from build123d import *

# Parameters (mm, degrees)
SKETCH_1_W                 = 50
SKETCH_1_H                 = 45
EXTRUDE_1_DEPTH            = 12
SHELL_1_T                  = -3
SHELL_1_THICKNESS_2_FACE_W = 39
SHELL_1_THICKNESS_2_FACE_H = 44
SHELL_1_THICKNESS_2_DEPTH  = 3
HOLE_WIZARD_1_AT_2_COUNT   = 2
HOLE_WIZARD_1_AT_2_PITCH   = 35
HOLE_WIZARD_1_AT_3_COUNT   = 2
HOLE_WIZARD_1_AT_3_PITCH   = 46.097722286
HOLE_WIZARD_1_AT_4_COUNT   = 2
HOLE_WIZARD_1_AT_4_PITCH   = 30
CUT_EXTRUDE_START          = -40
SKETCH_4_W                 = 18
SKETCH_4_H                 = 6
CUT_EXTRUDE_1_DEPTH        = 12
SKETCH_5_W                 = 44
SKETCH_5_H                 = 6
CUT_EXTRUDE_2_DEPTH        = 12
SKETCH_6_W                 = 26
SKETCH_6_H                 = 12
CUT_EXTRUDE_3_DEPTH        = 12


with BuildPart() as part:
    # 草图1 → 凸台-拉伸1 (new body)
    with BuildSketch(Plane(origin=(0, 0, 0), x_dir=(1, 0, 0), z_dir=(0, 1, 0))):
        Rectangle(SKETCH_1_W, SKETCH_1_H)
    extrude(amount=EXTRUDE_1_DEPTH)

    # 抽壳1
    shell_1_openings = [part.faces().sort_by_distance(p)[0] for p in [
        (0, 12, 0),
    ]]
    offset(amount=SHELL_1_T, openings=shell_1_openings, kind=Kind.INTERSECTION)

    # 抽壳1 thickness 2 face (on inner face of the shell) → 抽壳1 thickness 2 (add)
    with BuildSketch(Plane(origin=(0, 3, 0), x_dir=(0, 0, -1), z_dir=(0, -1, 0))):
        Rectangle(SHELL_1_THICKNESS_2_FACE_W, SHELL_1_THICKNESS_2_FACE_H)
    extrude(amount=-SHELL_1_THICKNESS_2_DEPTH)

    # 草图3 → 打孔尺寸(%根据)内六角圆柱头螺钉的类型1 (revolve, cut)
    with BuildSketch(Plane(origin=(-17.5, 0, 15), x_dir=(0, 0, -1), z_dir=(1, 0, 0))):
        Polygon((0, 0), (0, 12), (1.8, 12), (1.8, 3.4), (3, 3.4), (3, 0.025), (3.025, 0), align=None)
    hole_wizard_1 = revolve(axis=Axis((-17.5, -6.35, 15), (0, 1, 0)), mode=Mode.SUBTRACT)

    # 打孔尺寸(%根据)内六角圆柱头螺钉的类型1 at 2: 打孔尺寸(%根据)内六角圆柱头螺钉的类型1 ×2
    with Locations(*[(i * HOLE_WIZARD_1_AT_2_PITCH, 0, 0) for i in range(1, HOLE_WIZARD_1_AT_2_COUNT)]):
        add(hole_wizard_1, mode=Mode.SUBTRACT)

    # 打孔尺寸(%根据)内六角圆柱头螺钉的类型1 at 3: 打孔尺寸(%根据)内六角圆柱头螺钉的类型1 ×2
    with Locations(*[Vector(0.7592566023652966, 0, -0.6507913734559685) * (i * HOLE_WIZARD_1_AT_3_PITCH) for i in range(1, HOLE_WIZARD_1_AT_3_COUNT)]):
        add(hole_wizard_1, mode=Mode.SUBTRACT)

    # 打孔尺寸(%根据)内六角圆柱头螺钉的类型1 at 4: 打孔尺寸(%根据)内六角圆柱头螺钉的类型1 ×2
    with Locations(*[(0, 0, -i * HOLE_WIZARD_1_AT_4_PITCH) for i in range(1, HOLE_WIZARD_1_AT_4_COUNT)]):
        add(hole_wizard_1, mode=Mode.SUBTRACT)

    # 草图4 → 切除-拉伸1 (cut)
    with BuildSketch(Plane.XY.offset(22.5).offset(CUT_EXTRUDE_START)):
        with Locations((4, 9)):
            Rectangle(SKETCH_4_W, SKETCH_4_H)
    extrude(amount=-CUT_EXTRUDE_1_DEPTH, mode=Mode.SUBTRACT)

    # 草图5 → 切除-拉伸2 (cut)
    with BuildSketch(Plane.XY.offset(22.5)):
        with Locations((0, 9)):
            Rectangle(SKETCH_5_W, SKETCH_5_H)
    extrude(amount=-CUT_EXTRUDE_2_DEPTH, mode=Mode.SUBTRACT)

    # 草图6 → 切除-拉伸3 (cut)
    with BuildSketch(Plane(origin=(0, 6, 0), x_dir=(1, 0, 0), z_dir=(0, 1, 0))):
        with Locations((-9, -16.5)):
            Rectangle(SKETCH_6_W, SKETCH_6_H)
    extrude(amount=-CUT_EXTRUDE_3_DEPTH, mode=Mode.SUBTRACT)


solid = part.part
Can you work these out from the model? Positions are in its coordinate system, mm. A direction names the side the tool comes from. Give positions to 0.01 mm unless a question says otherwise; leave off trailing zeros. Loops run counter-clockwise (first coordinate to the right, second up) from the corner with the lowest first, then second, coordinate; pieces in that order, holes last. Notation, with made-up numbers: (70.25, 28) -> (96.25, 28) arc R13 cw to (96.25, 45) -> close; hole circle Ø1 at (24.5, -25). An arc over 180 degrees is marked (long way). Return JSON: item names as keys, results as strings.
Q1. I want a section at B-B, the plane z = 15. List the corners of the cut face in (x, y) for me (3 decimals).
Checks:
{"outline": "(-25, 0) -> (-22, 0) -> (-22, 12) -> (-25, 12) -> close; (4, 0) -> (14.475, 0) -> (14.5, 0.025) -> (14.5, 3.4) -> (15.7, 3.4) -> (15.7, 6) -> (4, 6) -> close; (19.3, 3.4) -> (20.5, 3.4) -> (20.5, 0.025) -> (20.525, 0) -> (25, 0) -> (25, 12) -> (22, 12) -> (22, 6) -> (19.3, 6) -> close"}
Q2. I need wall thicknesses on probe 1 along Z at (x, y) = (17.5, 5.5); probe 2 along X at (y, z) = (4.85, -15); probe 3 along Z at (x, y) = (17.5, 1.5). Which ranges of each line are inside material? Lowest first, please.
Checks:
{"probe 1": "z = -22.5 to -16.8, -13.2 to 13.2, 16.8 to 22.5", "probe 2": "x = -25 to -19.3, -15.7 to 15.7, 19.3 to 25", "probe 3": "z = -22.5 to -18, -12 to 12, 18 to 22.5"}
Q3. On a 3-axis mill with a long thin cutter (end or side, diameter ignored), from which of +Z, -Z, +X, -X, +Y, -Y can I reach the whole of each face in a straight line? I mean faces 4 (the face through (-15.7, 1.7, -12.6)), 5 (the face through (13, 9, -21)), 6 (the face through (-22.5, 12, -5.1)), 7 (the face through (4, 3, 17)), 8 (the face through (-22, 7, 6)). Say none if no direction works.
Checks:
{"face 4": "-Y", "face 5": "+Z, -Z, +Y", "face 6": "+Z, -Z, +X, -X, +Y", "face 7": "+Z, +Y, -Y", "face 8": "+Z, +Y"}
Q4. For pin 1 Ø5.5 at (x, z) = (17.5, -15) entering from -Y; pin 2 Ø8 at (x, z) = (0, 1.5) entering from +Y; pin 3 Ø1.8 at (x, y) = (-13, 3.5) entering from +Z; pin 4 Ø3 at (x, z) = (17.5, 15) entering from -Y, each with a flat end and sliding along its axis, tell me the tip position at first contact or that it passes through.
Checks:
{"pin 1": "stops at y = 3.4", "pin 2": "stops at y = 6", "pin 3": "stops at z = 10.5", "pin 4": "passes through"}
Q5. We'd pull the mould along Z, two halves only. Please class faces 1 (the face through (17, 9, -19.5)), 2 (the face through (19.5, 3.4, 15)), 3 (the face through (25, 6, 0)): released by +Z, released by -Z, zero draft, split by the parting line, or undercut.
Checks:
{"face 1": "released by +Z", "face 2": "undercut", "face 3": "zero draft"}
Q6. I want a section at A-A, the plane x = -17.5. List the corners of the cut face in (y, z) for me (3 decimals), then the cut area to 3 significant figures.
Checks:
{"outline": "(0, -22.5) -> (12, -22.5) -> (12, -19.5) -> (6, -19.5) -> (6, -16.8) -> (3.4, -16.8) -> (3.4, -18) -> (0.025, -18) -> (0, -18.025) -> close; (0, -11.975) -> (0.025, -12) -> (3.4, -12) -> (3.4, -13.2) -> (6, -13.2) -> (6, 10.5) -> (0, 10.5) -> close", "area": "186 mm2"}
Q7. I want a section at D-D, the plane x = 17.5. List the corners of the cut face in (y, z) for me (3 decimals).
Checks:
{"outline": "(0, -22.5) -> (12, -22.5) -> (12, -19.5) -> (6, -19.5) -> (6, -16.8) -> (3.4, -16.8) -> (3.4, -18) -> (0.025, -18) -> (0, -18.025) -> close; (0, -11.975) -> (0.025, -12) -> (3.4, -12) -> (3.4, -13.2) -> (6, -13.2) -> (6, 13.2) -> (3.4, 13.2) -> (3.4, 12) -> (0.025, 12) -> (0, 11.975) -> close; (0, 18.025) -> (0.025, 18) -> (3.4, 18) -> (3.4, 16.8) -> (6, 16.8) -> (6, 22.5) -> (0, 22.5) -> close"}
Q8. I want a section at C-C, the plane y = 9. List the corners of the cut face in (x, z) for me, then the cut area to 3 significant figures.
Checks:
{"outline": "(-25, -22.5) -> (-5, -22.5) -> (-5, -19.5) -> (-22, -19.5) -> (-22, 22.5) -> (-25, 22.5) -> close; (13, -22.5) -> (25, -22.5) -> (25, 22.5) -> (22, 22.5) -> (22, -19.5) -> (13, -19.5) -> close", "area": "348 mm2"}
